CAD build for the part. Positions are in the model's coordinates, mm. A direction names the side the tool comes from. Round coordinates to 2 decimals unless told otherwise and drop trailing zeros. Order: outer loops, then holes, each group sorted by start corner. A loop starts at its lowest first (then second) coordinate and runs counter-clockwise, first axis right, second up. Notation, with made-up numbers: (-20.5, 45) - (22.5, 45) arc R13 cw to (22.5, 60) - close; hole circle Ø1 at (68.5, -21.75). An arc over 180 degrees is marked (long way). Write item = value, one per line.
from build123d import *

# Parameters (mm, degrees)
F1_DEPTH = 25
F2_R     = 5
F3_R     = 4.99999
F4_R     = 4.99999


# Not quite as in the source:
# - a fillet or chamfer is up to 0.001 mm smaller than in the source, because OpenCascade refuses the exact size


with BuildPart() as f1:
    # F0 (on Top) → F1 (new body)
    with BuildSketch(Plane.XY):
        with BuildLine():
            Line((-4.1666666667, 24.6503324296), (-62.5, 14.7901994577))
            ThreePointArc((-62.5, 14.7901994577), (-75, 0), (-62.5, -14.7901994577))
            Line((-62.5, -14.7901994577), (-4.1666666667, -24.6503324296))
            ThreePointArc((-4.1666666667, -24.6503324296), (25, 0), (-4.1666666667, 24.6503324296))
        make_face()
        with BuildLine():
            Line((-60.8333333333, 4.9300664859), (-2.5, 14.7901994577))
            ThreePointArc((-2.5, 14.7901994577), (15, 0), (-2.5, -14.7901994577))
            Line((-2.5, -14.7901994577), (-60.8333333333, -4.9300664859))
            ThreePointArc((-60.8333333333, -4.9300664859), (-65, 0), (-60.8333333333, 4.9300664859))
        make_face(mode=Mode.SUBTRACT)
    extrude(amount=F1_DEPTH)

    # F2
    f2_edges = [f1.edges().sort_by_distance(p)[0] for p in [
        (-33.333333, -19.720266, 25),
        (25, 0, 25),
        (-33.333333, -19.720266, 0),
        (25, 0, 0),
    ]]
    fillet(f2_edges, radius=F2_R)

    # F3 (radius 5 in the source; OpenCascade refuses exactly that, so slightly less here)
    f3_edges = [f1.edges().sort_by_distance(p)[0] for p in [
        (-31.666667, 9.860133, 25),
    ]]
    fillet(f3_edges, radius=F3_R)

    # F4 (radius 5 in the source; OpenCascade refuses exactly that, so slightly less here)
    f4_edges = [f1.edges().sort_by_distance(p)[0] for p in [
        (15, 0, 0),
        (-31.666667, 9.860133, 0),
    ]]
    fillet(f4_edges, radius=F4_R)


solid = f1.part
(1) Band-saw the part on B-B on z = 22.5. List the corners of the cut face in (x, y).
Solved:
outline = (-62.39, -14.13) - (-4.06, -23.99) arc R24.33 ccw (long way) to (-4.06, 23.99) - (-62.39, 14.13) arc R14.33 ccw to start; hole (-60.94, -5.59) - (-2.61, -15.45) arc R15.67 ccw (long way) to (-2.61, 15.45) - (-60.94, 5.59) arc R5.67 ccw to start
(2) Drop flat-ended pins along their axis: pin 1 (2 mm diameter, centred on x = -24.5, z = 21, fed in from +Y); pin 2 (10 mm diameter, centred on y = -16.5, z = 20, fed in from -X); pin 3 (3 mm diameter, centred on x = 13.5, y = 17, fed in from +Z); pin 4 (8 mm diameter, centred on x = -60.5, y = -12, fed in from -Z). Give the stop position or say it passes through.
Solved:
pin_1 = 21.33
pin_2 = -69.63
pin_3 = 25
pin_4 = 0
(3) Tool access for faces 1 (the cylindrical face through (-32.33, -11.27, 23.57)), 2 (the cylindrical face through (-31.5, 11.34, 1.5)), 3 (the flat face through (-32.07, 9.79, 12.39)), 4 (the cylindrical face through (-75, 0, 12)): list every direction of +Z, -Z, +X, -X, +Y, -Y with a clear straight run to the whole face (end or side of a thin tool).
Solved:
face_1 = +Z
face_2 = -Z
face_3 = +Z, -Z
face_4 = +Z, -Z, -X
(4) Pull direction X, two halves, no side cores. Call faces 5 (the cylindrical face through (-32.69, -18.38, 23.5)), 6 (the flat face through (-31.26, -9.93, 12.39)): released by +X, released by -X, zero draft, split by the parting line, or undercut.
Solved:
face_5 = released by -X
face_6 = undercut
(5) Probe line 1 along Y through (x, z) = (0, 8.75); line 2 along Y through (x, z) = (9.5, 16.5); line 3 along X through (y, z) = (1.5, 15.25). List the from-to ranges inside material, lowest first.
Solved:
line_1 = -25 to -15, 15 to 25
line_2 = -23.12 to -11.61, 11.61 to 23.12
line_3 = -74.92 to -64.77, 14.92 to 24.95
